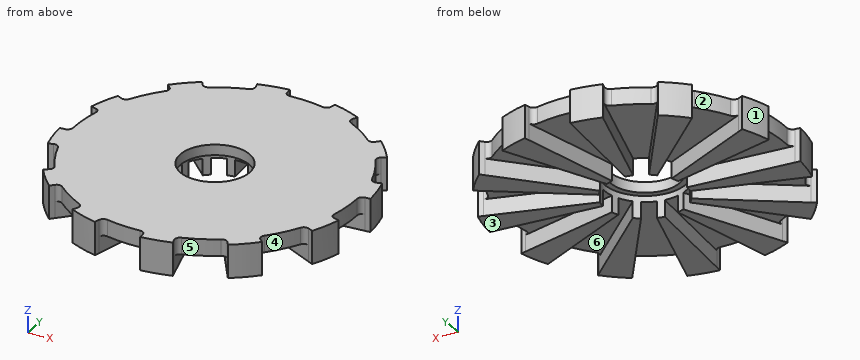
from build123d import *

# Parameters (mm, degrees)
CUT_EXTRUDE1_DEPTH = 125.362866242
CUT_EXTRUDE2_START = 9.525
CUT_EXTRUDE2_DEPTH = 9.525
CIRPATTERN2_COUNT  = 12


with BuildPart() as part:
    # Sketch4 → Revolve1 (revolve)
    with BuildSketch(Plane.YZ, mode=Mode.PRIVATE) as revolve1_sk:
        Polygon((-20, 19.05), (-86.9, 19.05), (-86.9, 0), (-23.5, 0), (-23.5, 13), (-20, 13), align=None)
    revolve(revolve1_sk.sketch.rotate(Axis((0, 0, 0), (0, 0, 1)), 270), axis=Axis((0, 0, 0), (0, 0, 1)))

    # Sketch1_4 → Cut-Extrude1 (cut, symmetric)
    with BuildSketch(Plane(origin=(0, 0, 0), x_dir=(0, 1, 0), z_dir=(0, 0, 1))):
        with BuildLine():
            ThreePointArc((-26.597315924, 82.729636683), (-22.823082808, 80.79181203), (-24.76090746, 77.017578914))
            ThreePointArc((-24.76090746, 77.017578914), (-34.189817375, 73.320299971), (-43.08288383, 68.47390102))
            ThreePointArc((-43.08288383, 68.47390102), (-47.219723812, 69.415471497), (-46.278153335, 73.552311479))
            ThreePointArc((-46.278153335, 73.552311479), (-36.725526945, 78.758146693), (-26.597315924, 82.729636683))
        make_face()
        with BuildLine():
            ThreePointArc((-46.278153335, 73.552311479), (-47.580918493, 72.716340635), (-48.868586739, 71.857297682))
            Line((-48.868586739, 71.857297682), (-47.16763138, 69.335527658))
            ThreePointArc((-47.16763138, 69.335527658), (-47.615924361, 71.632293551), (-46.278153335, 73.552311479))
        make_face()
        with BuildLine():
            ThreePointArc((-23.633761528, 83.62448993), (-25.119523803, 83.190260992), (-26.597315924, 82.729636683))
            ThreePointArc((-26.597315924, 82.729636683), (-24.26659404, 82.520264913), (-22.795326532, 80.700519613))
            Line((-22.795326532, 80.700519613), (-23.633761528, 83.62448993))
        make_face()
    cut_extrude1 = extrude(amount=CUT_EXTRUDE1_DEPTH, both=True, mode=Mode.SUBTRACT)

    # Sketch1 → Cut-Extrude2 (cut)
    with BuildSketch(Plane(origin=(0, 0, 0), x_dir=(0, 1, 0), z_dir=(0, 0, 1)).offset(CUT_EXTRUDE2_START)):
        with BuildLine():
            ThreePointArc((-43.08288383, 68.47390102), (-45.299705883, 68.077700471), (-47.16763138, 69.335527658))
            Line((-47.16763138, 69.335527658), (-10.3132812, 14.696706561))
            ThreePointArc((-10.3132812, 14.696706561), (-6.339273926, 13.594616806), (-4.629081023, 17.347292634))
            Line((-4.629081023, 17.347292634), (-22.795326532, 80.700519613))
            ThreePointArc((-22.795326532, 80.700519613), (-23.032454577, 78.461090147), (-24.76090746, 77.017578914))
            ThreePointArc((-24.76090746, 77.017578914), (-34.189817375, 73.320299971), (-43.08288383, 68.47390102))
        make_face()
    cut_extrude2 = extrude(amount=-CUT_EXTRUDE2_DEPTH, mode=Mode.SUBTRACT)

    # CirPattern2: Cut-Extrude1, Cut-Extrude2 ×12 about axis
    cirpattern2_axis = Axis((0, 0, 0), (0, 0, 1))
    add([cut_extrude1.rotate(cirpattern2_axis, i * 360 / CIRPATTERN2_COUNT) for i in range(1, CIRPATTERN2_COUNT)], mode=Mode.SUBTRACT)
    add([cut_extrude2.rotate(cirpattern2_axis, i * 360 / CIRPATTERN2_COUNT) for i in range(1, CIRPATTERN2_COUNT)], mode=Mode.SUBTRACT)


solid = part.part
Work out the finished part from the listing and answer in its coordinate system (mm). Face numbers are marked on the shaded views. A direction names the side the tool comes from. Coordinates: 2 decimals unless noted, no trailing zeros. Order: outer loops, then holes, each group sorted by start corner. A loop starts at its lowest first (then second) coordinate and runs counter-clockwise, first axis right, second up. Notation, with made-up numbers: (50.5, 0.5) - (68.5, 0.5) arc R8 ccw to (68.5, 10.5) - close; hole circle Ø10 at (83.5, -10). An arc over 180 degrees is marked (long way). Put each result on its own line as item: value. Start each with the question number.
1) Find section B-B (z = 2). State how many separate pieces and enclosed holes the cut face has, plus the area to 3 significant figures.
2) Find section D-D (x = 33). Give the vertices of the cut face in (y, z) (3 decimals).
3) Find section A-A (x = 0). Give the vertices of the cut face in (y, z) (3 decimals), plus the area to 3 significant figures.
4) For a pull along Y with two mould halves and no side action, classify the marked faces 1, 2 and 3 as released by +Y, released by -Y, zero draft, split by the parting line, or undercut.
5) Flat-ended cylindrical pins translate along their axes: pin 1 (10 mm diameter, centred on x = 29.5, z = 2.5, fed in from -Y) (3 decimals); pin 2 (4 mm diameter, centred on x = 62.5, z = 10.5, fed in from +Y); pin 3 (6 mm diameter, centred on x = 53, z = 14.5, fed in from -Y). Find the tip coordinate at first contact, or state that the pin passes through.
6) For the marked faces 4, 5 and 6, determine the directions among +Z, -Z, +X, -X, +Y, -Y from which every point of the face is accessible in a straight line to the end or side of a thin tool.
7) Find section C-C (y = -40). Give the vertices of the cut face in (x, z) (3 decimals), plus the area to 3 significant figures.
8) Find the intervals of material crossed by line 1 (X direction, y = -30.5, z = 2.5); line 2 (Y direction, x = 45, z = 2); line 3 (Y direction, x = 0, z = 14.5), in increasing order. Write a range as from..to.
Results list:
1. separate pieces: 12
1. enclosed holes: 0
1. area: 8,290 mm^2
2. outline: (-73.863, 9.525) - (-48.331, 9.525) - (-48.331, 0) - (-32.329, 0) - (-32.329, 9.525) - (-15.726, 9.525) - (-15.726, 0) - (-8.57, 0) - (-8.57, 9.525) - (2.64, 9.525) - (2.64, 0) - (9.117, 0) - (9.117, 9.525) - (22.659, 9.525) - (22.659, 0) - (33.695, 0) - (33.695, 9.525) - (68.417, 9.525) - (68.417, 0) - (80.39, 0) - (80.39, 19.05) - (-73.863, 19.05) - close
3. outline: (-80.9, 9.525) - (-23.5, 9.525) - (-23.5, 13) - (-20, 13) - (-20, 19.05) - (-80.9, 19.05) - close; (20, 13) - (23.5, 13) - (23.5, 9.525) - (80.9, 9.525) - (80.9, 19.05) - (20, 19.05) - close
3. area: 1,140 mm^2
4. face 1: released by +Y
4. face 2: undercut
4. face 3: zero draft
5. pin 1: stops at y = -50.555
5. pin 2: stops at y = 62.28
5. pin 3: stops at y = -71.07
6. face 4: +Z, -Z, +X
6. face 5: +Z, -Z, -Y
6. face 6: -Z
7. outline: (-70.319, 9.525) - (-58.709, 9.525) - (-58.709, 0) - (-39.089, 0) - (-39.089, 9.525) - (-19.14, 9.525) - (-19.14, 0) - (-10.315, 0) - (-10.315, 9.525) - (3.13, 9.525) - (3.13, 0) - (11.125, 0) - (11.125, 9.525) - (27.381, 9.525) - (27.381, 0) - (40.944, 0) - (40.944, 9.525) - (70.319, 9.525) - (70.319, 19.05) - (-70.319, 19.05) - close
7. area: 1,820 mm^2
8. line 1: x = -44.62..-29.91, -14.51..-7.95, 2.47..8.4, 20.97..31.11, 63.29..81.37
8. line 2: y = -66.12..-43.92, -21.58..-11.56, 3.48..12.56, 30.75..46.12
8. line 3: y = -80.9..-20, 20..80.9
